from build123d import *

# Parameters (mm, degrees)
SKETCH1_W           = 20
SKETCH1_H           = 30
BOSS_EXTRUDE1_DEPTH = 3
SKETCH2_W           = 5
SKETCH2_H           = 30
BOSS_EXTRUDE2_DEPTH = 10
SKETCH3_R           = 1.5
CUT_EXTRUDE1_DEPTH  = 10
SKETCH4_R           = 1.5
CUT_EXTRUDE2_DEPTH  = 4


with BuildPart() as part:
    # Sketch1 → Boss-Extrude1 (new body)
    with BuildSketch(Plane(origin=(0, 0, 0), x_dir=(1, 0, 0), z_dir=(0, 1, 0))):
        Rectangle(SKETCH1_W, SKETCH1_H)
    extrude(amount=BOSS_EXTRUDE1_DEPTH)

    # Sketch2 → Boss-Extrude2 (add)
    with BuildSketch(Plane(origin=(0, 3, 0), x_dir=(1, 0, 0), z_dir=(0, 1, 0))):
        with Locations((-7.5, 0)):
            Rectangle(SKETCH2_W, SKETCH2_H)
    extrude(amount=BOSS_EXTRUDE2_DEPTH)

    # Sketch3 → Cut-Extrude1 (cut)
    with BuildSketch(Plane.ZY.offset(10)):
        with Locations((10, 7)):
            Circle(SKETCH3_R)
    extrude(amount=-CUT_EXTRUDE1_DEPTH, mode=Mode.SUBTRACT)

    # Sketch4 → Cut-Extrude2 (cut, through all)
    with BuildSketch(Plane(origin=(0, 3, 0), x_dir=(1, 0, 0), z_dir=(0, 1, 0))):
        with Locations((2.5, -7.5)):
            Circle(SKETCH4_R)
        with Locations((2.5, 7.5)):
            Circle(SKETCH4_R)
    extrude(amount=-CUT_EXTRUDE2_DEPTH, mode=Mode.SUBTRACT)


solid = part.part
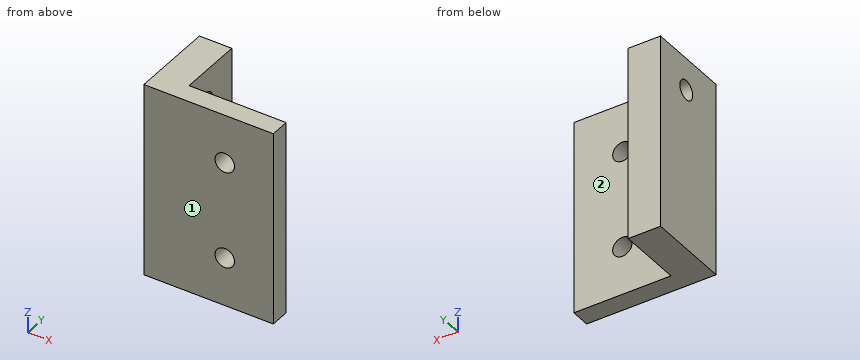
Verification items for the finished model (mm, model axes). Face numbers are marked on the shaded views. A direction names the side the tool comes from. Round coordinates to 2 decimals unless told otherwise and drop trailing zeros. Order: outer loops, then holes, each group sorted by start corner. A loop starts at its lowest first (then second) coordinate and runs counter-clockwise, first axis right, second up. Notation, with made-up numbers: (84.25, -34.75) -> (103.25, -34.75) arc R14 ccw to (103.25, -14.75) -> close; hole circle Ø10 at (28, 47). An arc over 180 degrees is marked (long way). Put each result on its own line as item: value.
1) Depth check by flat-ended pin: pin 1 (2 mm diameter, centred on y = 8.5, z = 11.5, fed in from +X); pin 2 (12 mm diameter, centred on x = -7.5, z = -5, fed in from -Y); pin 3 (12 mm diameter, centred on x = 5, z = 4.5, fed in from +Y). Enter the tip coordinate at first touch or a pass-through.
Final values:
pin 1: stops at x = -5
pin 2: stops at y = 0
pin 3: stops at y = 3
2) Section check A-A (z = -7.5). Record the cut outline in (x, y).
Final values:
outline: (-10, 0) -> (1, 0) -> (1, 3) -> (-5, 3) -> (-5, 13) -> (-10, 13) -> close; (4, 0) -> (10, 0) -> (10, 3) -> (4, 3) -> close
3) Set-up check for the marked faces 1 and 2: record each of +Z, -Z, +X, -X, +Y, -Y from which the full face is reachable in a straight line by a thin tool's end or side.
Final values:
face 1: +Z, -Z, +X, -X, -Y
face 2: +Z, -Z, +X, +Y
4) Material ranges on line 1 (Z direction, x = 2.5, y = 1.05); line 2 (X direction, y = 1.55, z = -7.5); line 3 (Y direction, x = -8.9, z = 10), recorded low to high.
Final values:
line 1: z = -15 to -9, -6 to 6, 9 to 15
line 2: x = -10 to 1, 4 to 10
line 3: y = 0 to 5.5, 8.5 to 13
5) Section check C-C (z = 10). Record the cut outline in (x, y), then the cut area to 3 significant figures.
Final values:
outline: (-10, 0) -> (10, 0) -> (10, 3) -> (-5, 3) -> (-5, 5.5) -> (-10, 5.5) -> close; (-10, 8.5) -> (-5, 8.5) -> (-5, 13) -> (-10, 13) -> close
area: 95.0 mm^2
6) Section check D-D (z = 2.25). Record the cut outline in (x, y), then the cut area to 3 significant figures.
Final values:
outline: (-10, 0) -> (10, 0) -> (10, 3) -> (-5, 3) -> (-5, 13) -> (-10, 13) -> close
area: 110 mm^2
7) Section check B-B (x = -7.5). Record the cut outline in (y, z).
Final values:
outline: (0, -15) -> (13, -15) -> (13, 15) -> (0, 15) -> close; hole circle Ø3 at (7, 10)
